```python
from build123d import *

# Parameters (mm, degrees)
SKETCH1_W           = 50
SKETCH1_H           = 20
BOSS_EXTRUDE1_DEPTH = 40
SKETCH2_W           = 18.2
SKETCH2_H           = 16.2
CUT_EXTRUDE1_DEPTH  = 4
CUT_EXTRUDE2_START  = -16
SKETCH3_R           = 2.5
CUT_EXTRUDE2_DEPTH  = 15
CUT_EXTRUDE3_DEPTH  = 1
CUT_EXTRUDE4_DEPTH  = 12
SKETCH7_W           = 18.2
SKETCH7_H           = 16.2
BOSS_EXTRUDE3_DEPTH = 1.5
CUT_EXTRUDE5_REACH  = 53.235
SKETCH8_R           = 1


with BuildPart() as part:
    # Sketch1 → Boss-Extrude1 (new, symmetric)
    with BuildSketch(Plane.XY):
        Rectangle(SKETCH1_W, SKETCH1_H)
    extrude(amount=BOSS_EXTRUDE1_DEPTH, both=True)

    # Sketch2 → Cut-Extrude1 (cut)
    with BuildSketch(Plane(origin=(0, 10, 0), x_dir=(1, 0, 0), z_dir=(0, 1, 0))):
        with Locations((0, 28.1)):
            Rectangle(SKETCH2_W, SKETCH2_H)
    extrude(amount=-CUT_EXTRUDE1_DEPTH, mode=Mode.SUBTRACT)

    # Sketch3 → Cut-Extrude2 (cut)
    with BuildSketch(Plane(origin=(0, 6, 0), x_dir=(1, 0, 0), z_dir=(0, 1, 0)).offset(CUT_EXTRUDE2_START)):
        with Locations(Location((-5.1, 32.2, 0), (0, 0, 180))):
            Circle(SKETCH3_R)
        with Locations(Location((0.1, 32.2, 0), (0, 0, 180))):
            Circle(SKETCH3_R)
        with Locations(Location((-3.1, 24, 0), (0, 0, 180))):
            Circle(SKETCH3_R)
        with Locations(Location((2.1, 24, 0), (0, 0, 180))):
            Circle(SKETCH3_R)
    extrude(amount=CUT_EXTRUDE2_DEPTH, mode=Mode.SUBTRACT)

    # Sketch4 → Cut-Extrude3 (cut)
    with BuildSketch(Plane(origin=(0, 6, 0), x_dir=(1, 0, 0), z_dir=(0, 1, 0))):
        Polygon((-5.5, 33.824807681), (-7, 33.824807681), (-7, 30.575192319), (-5.5, 30.575192319), (-5.5, 30.828384848), (-4.7, 30.828384848), (-4.7, 30.575192319), (-3.2, 30.575192319), (-3.2, 33.824807681), (-4.7, 33.824807681), (-4.7, 33.571615152), (-5.5, 33.571615152), align=None)
        Polygon((0.5, 30.575192319), (0.5, 30.828384848), (-0.3, 30.828384848), (-0.3, 30.575192319), (-1.8, 30.575192319), (-1.8, 33.824807681), (-0.3, 33.824807681), (-0.3, 33.571615152), (0.5, 33.571615152), (0.5, 33.824807681), (2, 33.824807681), (2, 30.575192319), align=None)
        Polygon((2.5, 22.375192325), (4.000000005, 22.375192325), (3.999999995, 25.624807687), (2.5, 25.624683497), (2.5, 25.371490969), (1.7, 25.371490983), (1.7, 25.624683512), (0.199999995, 25.624807675), (0.200000005, 22.375192313), (1.699999991, 22.37506815), (1.699999991, 22.628260678), (2.5, 22.628384854), align=None)
        Polygon((-3.5, 25.624683497), (-3.5, 25.371490969), (-2.7, 25.371490983), (-2.7, 25.624683512), (-1.199999995, 25.624807675), (-1.200000005, 22.375192313), (-2.699999991, 22.37506815), (-2.699999991, 22.628260678), (-3.5, 22.628384854), (-3.5, 22.375192325), (-5.000000005, 22.375192325), (-4.999999995, 25.624807687), align=None)
    extrude(amount=-CUT_EXTRUDE3_DEPTH, mode=Mode.SUBTRACT)

    # Sketch6 → Cut-Extrude4 (cut)
    with BuildSketch(Plane.XZ.offset(10)):
        Polygon((22.5, -36.2), (4, -36.2), (0, -36.2), (0, -29.2), (2.1, -29.2), (2.099999991, -20), (-3.1, -20), (-3.1, -29.2), (-5.1, -29.2), (-5.1, -36.2), (-9.1, -36.2), (-22.5, -36.2), (-22.5, 39), (22.5, 39), align=None)
    extrude(amount=-CUT_EXTRUDE4_DEPTH, mode=Mode.SUBTRACT)

    # Sketch7 → Boss-Extrude3 (add)
    with BuildSketch(Plane.XZ.offset(10)):
        with Locations((0, -28.1)):
            Rectangle(SKETCH7_W, SKETCH7_H)
    extrude(amount=-BOSS_EXTRUDE3_DEPTH)

    # Sketch8 → Cut-Extrude5 (cut, up to next)
    with BuildSketch(Plane.XZ.offset(10), mode=Mode.PRIVATE) as cut_extrude5_sk1:
        with Locations((-3.099999996, -24.000000006)):
            Circle(SKETCH8_R)
    cut_extrude5_tool1 = extrude(cut_extrude5_sk1.sketch, amount=-CUT_EXTRUDE5_REACH, mode=Mode.PRIVATE) & part.part
    # Sketch8 → Cut-Extrude5 (cut, up to next)
    with BuildSketch(Plane.XZ.offset(10), mode=Mode.PRIVATE) as cut_extrude5_sk2:
        with Locations((2.099999996, -24.000000006)):
            Circle(SKETCH8_R)
    cut_extrude5_tool2 = extrude(cut_extrude5_sk2.sketch, amount=-CUT_EXTRUDE5_REACH, mode=Mode.PRIVATE) & part.part
    # Sketch8 → Cut-Extrude5 (cut, up to next)
    with BuildSketch(Plane.XZ.offset(10), mode=Mode.PRIVATE) as cut_extrude5_sk3:
        with Locations((-5.1, -32.2)):
            Circle(SKETCH8_R)
    cut_extrude5_tool3 = extrude(cut_extrude5_sk3.sketch, amount=-CUT_EXTRUDE5_REACH, mode=Mode.PRIVATE) & part.part
    # Sketch8 → Cut-Extrude5 (cut, up to next)
    with BuildSketch(Plane.XZ.offset(10), mode=Mode.PRIVATE) as cut_extrude5_sk4:
        with Locations((0.1, -32.2)):
            Circle(SKETCH8_R)
    cut_extrude5_tool4 = extrude(cut_extrude5_sk4.sketch, amount=-CUT_EXTRUDE5_REACH, mode=Mode.PRIVATE) & part.part
    add(cut_extrude5_tool1.solids().sort_by_distance((-3.1, -10, -24))[0], mode=Mode.SUBTRACT)
    add(cut_extrude5_tool2.solids().sort_by_distance((2.1, -10, -24))[0], mode=Mode.SUBTRACT)
    add(cut_extrude5_tool3.solids().sort_by_distance((-5.1, -10, -32.2))[0], mode=Mode.SUBTRACT)
    add(cut_extrude5_tool4.solids().sort_by_distance((0.1, -10, -32.2))[0], mode=Mode.SUBTRACT)


solid = part.part
```
Work out the finished part from the listing and answer in its coordinate system (mm). A direction names the side the tool comes from. Coordinates: 2 decimals unless noted, no trailing zeros. Write each loop counter-clockwise with the first axis right and the second up, starting at its lowest first coordinate (ties: lowest second). Pieces come first, ordered by that corner, then holes.
Q1. A cutting plane is placed at A-A, the plane y = -4.75. Give the vertices of the cut face in (x, z), then the cut area to 3 significant figures.
Q2. Which of the six approach directions +Z, -Z, +X, -X, +Y, -Y give full straight-line access (tool end or side, diameter ignored) to faces 1 (the face through (0, 10, 1)), 2 (the face through (0, -4, 39)), 3 (the face through (9.1, 8, -28)), 4 (the face through (1, -3, -29.2))?
Q3. Determine the mould class of faces 5 (the face through (-25, 0, 1)), 6 (the face through (11, -4, -36.2)) for opening direction Z: released by +Z, released by -Z, zero draft, split by the parting line, or undercut.
Q4. Each of these flat-tipped pins is pushed along its axis until it touches: pin 1 Ø12 at (x, z) = (-4.5, 22.5) entering from -Y; pin 2 Ø3 at (x, z) = (-5.1, -32.2) entering from -Y; pin 3 Ø6 at (x, z) = (4.5, -29.5) entering from +Y. Where does it stop, or does it pass through?
Q5. A cutting plane is placed at C-C, the plane z = 25.5. Give the vertices of the cut face in (x, y).
Q6. Find the intervals of material crossed by line 1 (X direction, y = -1.75, z = -36); line 2 (X direction, y = 2.25, z = -32.2); line 3 (X direction, y = -9.6, z = -24), in increasing order.
Q7. A cutting plane is placed at B-B, the plane x = 13.5. Give the vertices of the cut face in (y, z), then the cut area to 3 significant figures.
Q8. A cutting plane is placed at D-D, the plane y = 8.75. Give the vertices of the cut face in (x, z), then the cut area to 3 significant figures.
Findings below:
1. outline: (-25, -40) - (25, -40) - (25, 40) - (-25, 40) - close; hole (-22.5, -36.2) - (-5.1, -36.2) - (-5.1, -34.7) arc R2.5 ccw to (-5.1, -29.7) - (-5.1, -29.2) - (-3.1, -29.2) - (-3.1, -26.5) arc R2.5 ccw to (-3.1, -21.5) - (-3.1, -20) - (2.1, -20) - (2.1, -21.5) arc R2.5 ccw to (2.1, -26.5) - (2.1, -29.2) - (0, -29.2) - (0, -29.7) arc R2.5 ccw to (0, -34.7) - (0, -36.2) - (22.5, -36.2) - (22.5, 39) - (-22.5, 39) - close
1. area: 661 mm2
2. face 1: +Z, -Z, +X, -X, +Y
2. face 2: -Y
2. face 3: +Y
2. face 4: none
3. face 5: zero draft
3. face 6: undercut
4. pin 1: stops at y = 2
4. pin 2: stops at y = -10
4. pin 3: stops at y = 6
5. outline: (-25, -10) - (-22.5, -10) - (-22.5, 2) - (22.5, 2) - (22.5, -10) - (25, -10) - (25, 10) - (-25, 10) - close
6. line 1: x = -25 to -22.5, -5.1 to 0, 22.5 to 25
6. line 2: x = -25 to -7.6, -2.6 to -2.4, 2.6 to 25
6. line 3: x = -25 to -22.5, -9.1 to -4.1, -2.1 to 1.1, 3.1 to 9.1, 22.5 to 25
7. outline: (-10, -40) - (10, -40) - (10, 40) - (-10, 40) - (-10, 39) - (2, 39) - (2, -36.2) - (-10, -36.2) - close
7. area: 698 mm2
8. outline: (-25, -40) - (25, -40) - (25, 40) - (-25, 40) - close; hole (-9.1, -36.2) - (9.1, -36.2) - (9.1, -20) - (-9.1, -20) - close
8. area: 3,710 mm2
